```python
from build123d import *

# Parameters (mm, degrees)
SKETCH1_R                       = 2.25
BOSS_EXTRUDE1_DEPTH             = 14
SKETCH2_W                       = 18
SKETCH2_H                       = 9.25
CUT_EXTRUDE1_DEPTH              = 24.849790355
BOSS_EXTRUDE2_DEPTH             = 2.6
BOSS_EXTRUDE2_DEPTH_BACK        = 2.6
SKETCH4_R                       = 2.25
BOSS_EXTRUDE3_DEPTH             = 28
SKETCH7_W                       = 4.5
SKETCH7_H                       = 3
CUT_EXTRUDE2_DEPTH              = 36.082738034
SKETCH9_W                       = 28
SKETCH9_H                       = 2
BOSS_EXTRUDE4_DEPTH             = 48
BOSS_EXTRUDE5_REACH             = 60.209
SKETCH11_W                      = 28
SKETCH11_H                      = 7.313537016
BOSS_EXTRUDE5_DIRECTION_2_REACH = 60.209
SKETCH14_R                      = 2.15
CUT_EXTRUDE6_DEPTH              = 59.208886884
SKETCH15_W                      = 48
SKETCH15_H                      = 2
SKETCH15_W_2                    = 7.313537016
SKETCH15_H_2                    = 13.819983601
CUT_EXTRUDE7_DEPTH              = 64.806460469
SKETCH16_W                      = 2
SKETCH16_H                      = 7
CUT_EXTRUDE8_DEPTH              = 32.608938609


with BuildPart() as part:
    # Sketch1 → Boss-Extrude1 (new, symmetric)
    with BuildSketch(Plane(origin=(0, 0, 0), x_dir=(0, 0, -1), z_dir=(1, 0, 0))):
        with BuildLine():
            Line((2.25, 1.5), (7.25, 1.5))
            Line((7.25, 1.5), (7.25, 8.5))
            Line((7.25, 8.5), (4.25, 8.5))
            ThreePointArc((4.25, 8.5), (0, 12.75), (-4.25, 8.5))
            Line((-4.25, 8.5), (-7.25, 8.5))
            Line((-7.25, 8.5), (-7.25, 1.5))
            Line((-7.25, 1.5), (-2.25, 1.5))
            Line((-2.25, 1.5), (-2.25, -1.5))
            Line((-2.25, -1.5), (2.25, -1.5))
            Line((2.25, -1.5), (2.25, 1.5))
        make_face()
        with Locations((0, 9)):
            Circle(SKETCH1_R, mode=Mode.SUBTRACT)
    extrude(amount=BOSS_EXTRUDE1_DEPTH, both=True)

    # Sketch2 → Cut-Extrude1 (cut, through all)
    with BuildSketch(Plane.XY.offset(7.25)):
        with Locations((0, 8.125)):
            Rectangle(SKETCH2_W, SKETCH2_H)
    extrude(amount=-CUT_EXTRUDE1_DEPTH, mode=Mode.SUBTRACT)

    # Sketch4 → Boss-Extrude2 (add, two sides: drawn at the far end of the back side and taken through both)
    with BuildSketch(Plane(origin=(0, 0, 0), x_dir=(0, 0, -1), z_dir=(1, 0, 0)).offset(-BOSS_EXTRUDE2_DEPTH_BACK)):
        with BuildLine():
            Line((-4.25, 8.5), (-7.25, 8.5))
            Line((-7.25, 8.5), (-7.25, 3.5))
            Line((-7.25, 3.5), (7.25, 3.5))
            Line((7.25, 3.5), (7.25, 8.5))
            Line((7.25, 8.5), (4.25, 8.5))
            ThreePointArc((4.25, 8.5), (0, 12.75), (-4.25, 8.5))
        make_face()
        with Locations(Location((0, 9, 0), (0, 0, 180))):
            Circle(SKETCH4_R, mode=Mode.SUBTRACT)
    extrude(amount=BOSS_EXTRUDE2_DEPTH + BOSS_EXTRUDE2_DEPTH_BACK)

    # Sketch6 → Boss-Extrude3 (add, through all)
    with BuildSketch(Plane.ZY.offset(14)):
        Polygon((7.25, 8.5), (14.563537016, 15.319983601), (14.563537016, 8.319983601), (7.25, 1.5), align=None)
    extrude(amount=-BOSS_EXTRUDE3_DEPTH)

    # Sketch7 → Cut-Extrude2 (cut, through all)
    with BuildSketch(Plane.ZY.offset(14)):
        Rectangle(SKETCH7_W, SKETCH7_H)
    extrude(amount=-CUT_EXTRUDE2_DEPTH, mode=Mode.SUBTRACT)

    # Sketch9 → Boss-Extrude4 (add)
    with BuildSketch(Plane(origin=(0, 0, -7.25), x_dir=(-1, 0, 0), z_dir=(0, 0, -1))):
        with Locations((0, 2.5)):
            Rectangle(SKETCH9_W, SKETCH9_H)
    extrude(amount=BOSS_EXTRUDE4_DEPTH)

    # Boss-Extrude5: up to this face of the body (flat: up to its plane)
    boss_extrude5_end = Plane(part.part.faces().sort_by_distance((0, 1.5, -24))[0])
    # Sketch11 → Boss-Extrude5 (add, up to the picked face)
    with BuildSketch(Plane(origin=(0, 3.5, 0), x_dir=(1, 0, 0), z_dir=(0, 1, 0)), mode=Mode.PRIVATE) as boss_extrude5_sk1:
        with Locations((0, -10.906768508)):
            Rectangle(SKETCH11_W, SKETCH11_H)
    boss_extrude5_tool1 = split(extrude(boss_extrude5_sk1.sketch, amount=-BOSS_EXTRUDE5_REACH, mode=Mode.PRIVATE), bisect_by=boss_extrude5_end, keep=Keep.BOTH, mode=Mode.PRIVATE)
    add(boss_extrude5_tool1.solids().sort_by(Axis((0, 3.5, 10.906769), (0, -1, 0)))[0])

    # Boss-Extrude5 direction 2: up to this face of the body (flat: up to its plane)
    boss_extrude5_direction_2_end = Plane(part.part.faces().sort_by_distance((0, 4.9099918, 10.906768508))[0])
    # Sketch11 → Boss-Extrude5 direction 2 (add, up to the picked face)
    with BuildSketch(Plane(origin=(0, 3.5, 0), x_dir=(1, 0, 0), z_dir=(0, 1, 0)), mode=Mode.PRIVATE) as boss_extrude5_direction_2_sk1:
        with Locations((0, -10.906768508)):
            Rectangle(SKETCH11_W, SKETCH11_H)
    boss_extrude5_direction_2_tool1 = split(extrude(boss_extrude5_direction_2_sk1.sketch, amount=BOSS_EXTRUDE5_DIRECTION_2_REACH, mode=Mode.PRIVATE), bisect_by=boss_extrude5_direction_2_end, keep=Keep.BOTH, mode=Mode.PRIVATE)
    add(boss_extrude5_direction_2_tool1.solids().sort_by(Axis((0, 3.5, 10.906769), (0, 1, 0)))[0])

    # Sketch14 → Cut-Extrude6 (cut, through all)
    with BuildSketch(Plane(origin=(0, 3.5, 0), x_dir=(1, 0, 0), z_dir=(0, 1, 0))):
        with Locations(Location((11, 51, 0), (0, 0, 270))):
            Circle(SKETCH14_R)
        with Locations(Location((11, 29, 0), (0, 0, 270))):
            Circle(SKETCH14_R)
        with Locations(Location((-11, 29, 0), (0, 0, 270))):
            Circle(SKETCH14_R)
        with Locations(Location((-11, 51, 0), (0, 0, 270))):
            Circle(SKETCH14_R)
    extrude(amount=-CUT_EXTRUDE6_DEPTH, mode=Mode.SUBTRACT)

    # Sketch15 → Cut-Extrude7 (cut, through all)
    with BuildSketch(Plane.ZY.offset(14)):
        with Locations((-31.25, 2.5)):
            Rectangle(SKETCH15_W, SKETCH15_H)
        with Locations((10.906768508, 8.409991801)):
            Rectangle(SKETCH15_W_2, SKETCH15_H_2)
    extrude(amount=-CUT_EXTRUDE7_DEPTH, mode=Mode.SUBTRACT)

    # Sketch16 → Cut-Extrude8 (cut, through all)
    with BuildSketch(Plane.ZY.offset(14)):
        with Locations((-6.25, 5)):
            Rectangle(SKETCH16_W, SKETCH16_H)
        with Locations((6.25, 5)):
            Rectangle(SKETCH16_W, SKETCH16_H)
    extrude(amount=-CUT_EXTRUDE8_DEPTH, mode=Mode.SUBTRACT)


solid = part.part
```
Could you check a few things on this model? Use its own coordinates, in mm. A direction names the side the tool comes from. Give positions to 0.01 mm unless a question says otherwise; leave off trailing zeros. Loops run counter-clockwise (first coordinate to the right, second up) from the corner with the lowest first, then second, coordinate; pieces in that order, holes last. Notation, with made-up numbers: (-15.75, -19.75) -> (39.25, -19.75) arc R26 ccw to (39.25, 8.25) -> close; hole circle Ø7 at (-10.75, 55). An arc over 180 degrees is marked (long way). Put each result on its own line as item: value.
(1) Please list where these lines run through material, in increasing order: probe 1 along X at (y, z) = (7.5, 2); probe 2 along Y at (x, z) = (0.65, 0); probe 3 along Z at (x, y) = (1.2, 9). Write a range as [from, to].
Computed:
probe 1: [-14, -9], [-2.6, 2.6], [9, 14]
probe 2: [1.5, 6.75], [11.25, 12.75]
probe 3: [-4.22, -2.25], [2.25, 4.22]
(2) Imagine slicing it at D-D on y = 9. Write out the boundary of the cut face in (x, z).
Computed:
outline: (-14, -4.22) -> (-9, -4.22) -> (-9, -2.25) -> (-14, -2.25) -> close; (-14, 2.25) -> (-9, 2.25) -> (-9, 4.22) -> (-14, 4.22) -> close; (-2.6, -4.22) -> (2.6, -4.22) -> (2.6, -2.25) -> (-2.6, -2.25) -> close; (-2.6, 2.25) -> (2.6, 2.25) -> (2.6, 4.22) -> (-2.6, 4.22) -> close; (9, -4.22) -> (14, -4.22) -> (14, -2.25) -> (9, -2.25) -> close; (9, 2.25) -> (14, 2.25) -> (14, 4.22) -> (9, 4.22) -> close
(3) I'm going to push flat-ended pins straight in: pin 1 Ø2.5 at (y, z) = (9, 0) entering from -X; pin 2 Ø0.5 at (x, z) = (0.5, 5) entering from +Y. Where does each tip first touch, or does it pass through?
Computed:
pin 1: through
pin 2: y = 8.5
(4) Imagine slicing it at A-A on y = 6.25. Write out the boundary of the cut face in (x, z), plus the area to 3 significant figures.
Computed:
outline: (-14, -5.25) -> (-9, -5.25) -> (-9, 5.25) -> (-14, 5.25) -> close; (-2.6, -5.25) -> (2.6, -5.25) -> (2.6, 5.25) -> (-2.6, 5.25) -> close; (9, -5.25) -> (14, -5.25) -> (14, 5.25) -> (9, 5.25) -> close
area: 160 mm^2
(5) Imagine slicing it at B-B on x = 0.75. Write out the boundary of the cut face in (y, z).
Computed:
outline: (1.5, -5.25) -> (8.5, -5.25) -> (8.5, -4.25) arc R4.25 ccw to (8.5, 4.25) -> (8.5, 5.25) -> (1.5, 5.25) -> close; hole circle Ø4.5 at (9, 0)
(6) For faces 1 (the face through (6, 3.5, 0)), 2 (the face through (0, 8.5, -5)), 3 (the face through (-11, 8.5, 5)), 4 (the face through (-0.04, 12.75, -0.09)), which set-ups out of +Z, -Z, +X, -X, +Y, -Y let a thin tool reach every point of the face, with its end or its side?
Computed:
face 1: +Z, -Z, +Y
face 2: -Z, +X, -X, +Y
face 3: +Z, +X, -X, +Y
face 4: +X, -X, +Y
(7) Thinking about a two-plate mould opening in X: for faces 5 (the face through (-6, 3.5, 0)), 6 (the face through (-0.04, 6.77, -0.29)), 7 (the face through (-14, 6, 0)), which applies, pulls with the +X half, pulls with the -X half, needs draft (parallel to the pull), parting line crosses it, or undercut?
Computed:
face 5: undercut
face 6: needs draft
face 7: pulls with the -X half
(8) Imagine slicing it at C-C on z = 0. Write out the boundary of the cut face in (x, y).
Computed:
outline: (-14, 1.5) -> (14, 1.5) -> (14, 6.75) -> (9, 6.75) -> (9, 3.5) -> (2.6, 3.5) -> (2.6, 6.75) -> (-2.6, 6.75) -> (-2.6, 3.5) -> (-9, 3.5) -> (-9, 6.75) -> (-14, 6.75) -> close; (-14, 11.25) -> (-9, 11.25) -> (-9, 12.75) -> (-14, 12.75) -> close; (-2.6, 11.25) -> (2.6, 11.25) -> (2.6, 12.75) -> (-2.6, 12.75) -> close; (9, 11.25) -> (14, 11.25) -> (14, 12.75) -> (9, 12.75) -> close
